from build123d import *

# Parameters (mm, degrees)
SKETCH_1_W          = 55
SKETCH_1_H          = 36.8
EXTRUDE_1_DEPTH     = 24
SKETCH_2_W          = 38
SKETCH_2_H          = 36.8
CUT_EXTRUDE_1_DEPTH = 1
CHAMFER_1_SIZE      = 0.5
CHAMFER_2_SIZE      = 0.5
SKETCH_3_W          = 7.5
SKETCH_3_H          = 36.8
CUT_EXTRUDE_2_DEPTH = 20
CHAMFER_3_SIZE      = 1.5
CHAMFER_4_SIZE      = 2
CHAMFER_5_SIZE      = 2
SKETCH_4_R          = 2.1
CUT_EXTRUDE_3_DEPTH = 20
SKETCH_5_R          = 5
EXTRUDE_2_DEPTH     = 10


with BuildPart() as part:
    # 草图1 → 凸台-拉伸1 (new body)
    with BuildSketch(Plane.XY):
        with Locations((-27.5, 18.4)):
            Rectangle(SKETCH_1_W, SKETCH_1_H)
    extrude(amount=EXTRUDE_1_DEPTH)

    # 草图2 → 切除-拉伸1 (cut)
    with BuildSketch(Plane.XY.offset(24)):
        with Locations((-27.5, 18.4)):
            Rectangle(SKETCH_2_W, SKETCH_2_H)
    extrude(amount=-CUT_EXTRUDE_1_DEPTH, mode=Mode.SUBTRACT)

    # 倒角1
    chamfer_1_edges = [part.edges().sort_by_distance(p)[0] for p in [
        (-46.5, 18.4, 24),
        (-8.5, 18.4, 24),
    ]]
    chamfer(chamfer_1_edges, length=CHAMFER_1_SIZE)

    # 倒角2
    chamfer_2_edges = [part.edges().sort_by_distance(p)[0] for p in [
        (-27.5, 36.8, 23),
        (-27.5, 0, 23),
    ]]
    chamfer(chamfer_2_edges, length=CHAMFER_2_SIZE)

    # 草图3 → 切除-拉伸2 (cut)
    with BuildSketch(Plane(origin=(0, 0, 0), x_dir=(-1, 0, 0), z_dir=(0, 0, -1))):
        with Locations((3.75, 18.4)):
            Rectangle(SKETCH_3_W, SKETCH_3_H)
        with Locations((51.25, 18.4)):
            Rectangle(SKETCH_3_W, SKETCH_3_H)
    extrude(amount=-CUT_EXTRUDE_2_DEPTH, mode=Mode.SUBTRACT)

    # 倒角3
    chamfer_3_edges = [part.edges().sort_by_distance(p)[0] for p in [
        (-27.5, 0, 0),
        (-27.5, 36.8, 0),
        (-7.5, 18.4, 0),
        (-47.5, 18.4, 0),
    ]]
    chamfer(chamfer_3_edges, length=CHAMFER_3_SIZE)

    # 倒角4
    chamfer_4_edges = [part.edges().sort_by_distance(p)[0] for p in [
        (-7.5, 36.8, 10.75),
        (-7.5, 0, 10.75),
        (-47.5, 0, 10.75),
        (-47.5, 36.8, 10.75),
    ]]
    chamfer(chamfer_4_edges, length=CHAMFER_4_SIZE)

    # 倒角5
    chamfer_5_edges = [part.edges().sort_by_distance(p)[0] for p in [
        (0, 0, 22),
        (-55, 0, 22),
        (-55, 36.8, 22),
        (0, 36.8, 22),
    ]]
    chamfer(chamfer_5_edges, length=CHAMFER_5_SIZE)

    # 草图4 → 切除-拉伸3 (cut)
    with BuildSketch(Plane(origin=(0, 0, 20), x_dir=(-1, 0, 0), z_dir=(0, 0, -1))):
        with Locations((3.55, 18.4)):
            Circle(SKETCH_4_R)
        with Locations((51.45, 32.75)):
            Circle(SKETCH_4_R)
        with Locations((51.45, 4.05)):
            Circle(SKETCH_4_R)
    extrude(amount=-CUT_EXTRUDE_3_DEPTH, mode=Mode.SUBTRACT)

    # 草图5 → 凸台-拉伸2 (add)
    with BuildSketch(Plane.ZY.offset(47.5)):
        with Locations(Location((10, 18.4, 0), (0, 0, 90))):
            Circle(SKETCH_5_R)
    extrude(amount=EXTRUDE_2_DEPTH)


solid = part.part
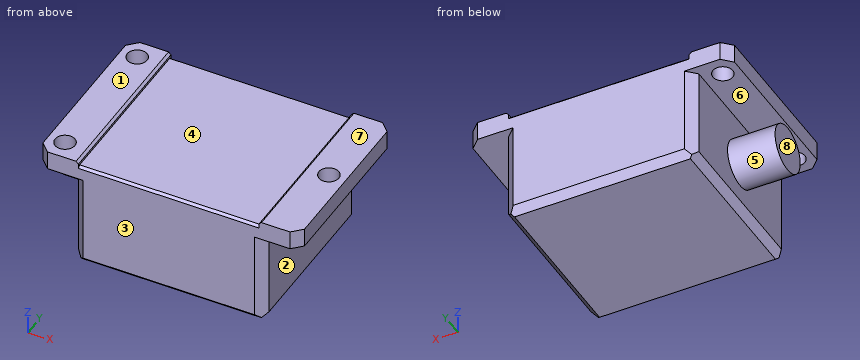
The listing builds one solid part. Answer for the finished solid, in the listing's coordinates (mm). Face numbers are marked on the shaded views. A direction names the side the tool comes from. Coordinates: 2 decimals unless noted, no trailing zeros. Loops run counter-clockwise (first coordinate to the right, second up) from the corner with the lowest first, then second, coordinate; pieces in that order, holes last. Notation, with made-up numbers: (8, -6) -> (14, -6) arc R18 cw to (14, 22) -> close; hole circle Ø1 at (-31, -35). An arc over 180 degrees is marked (long way). Answer in a Markdown table with one row per item. Add a question column.
1. The part is cut by section D-D, the plane y = 9.5. Write down the section's boundary in (x, z), then the cut area to 4 significant figures.
2. Determine the mould class of the marked faces 6, 7 and 8 for opening direction Z: +Z half, -Z half, draft (parallel to the pull), parting line (faces both ways), or undercut.
3. The part is cut by section A-A, the plane y = 18.4. Write down the section's boundary in (x, z).
4. Flat-ended cylindrical pins translate along their axes: P1, Ø4, axis at y = 18, z = 13, coming from the +X side; P2, Ø3, axis at y = 15.5, z = 21.5, coming from the -X side; P3, Ø1, axis at y = 8, z = 16.5, coming from the -X side; P4, Ø2.5, axis at x = -51.45, y = 4.05, coming from the +Z side. Find the tip coordinate at first contact, or state that the pin passes through.
5. For the marked faces 1, 2, 3, 4 and 5, determine the directions among +Z, -Z, +X, -X, +Y, -Y from which every point of the face is accessible in a straight line to the end or side of a thin tool.
6. Consider line 1 (Y direction, x = -3.55, z = 21.55); line 2 (Y direction, x = -51.45, z = 21.2); line 3 (Z direction, x = -13, y = 14). Determine where each line is inside the solid, lowest interval first. Write a range as [from, to].
7. The part is cut by section C-C, the plane x = -3.55. Write down the section's boundary in (y, z).
8. The part is cut by section B-B, the plane x = -51.45. Write down the section's boundary in (y, z), then the cut area to 3 significant figures.
Answer below:
| question | item | result |
|---|---|---|
| 1 | outline | (-55, 20) -> (-47.5, 20) -> (-47.5, 1.5) -> (-46, 0) -> (-9, 0) -> (-7.5, 1.5) -> (-7.5, 20) -> (0, 20) -> (0, 24) -> (-8, 24) -> (-8.5, 23.5) -> (-8.5, 23) -> (-46.5, 23) -> (-46.5, 23.5) -> (-47, 24) -> (-55, 24) -> close |
| 1 | area | 979.5 mm2 |
| 2 | face 6 | undercut |
| 2 | face 7 | +Z half |
| 2 | face 8 | draft |
| 3 | outline | (-57.5, 5) -> (-47.5, 5) -> (-47.5, 1.5) -> (-46, 0) -> (-9, 0) -> (-7.5, 1.5) -> (-7.5, 20) -> (-5.65, 20) -> (-5.65, 24) -> (-8, 24) -> (-8.5, 23.5) -> (-8.5, 23) -> (-46.5, 23) -> (-46.5, 23.5) -> (-47, 24) -> (-55, 24) -> (-55, 20) -> (-47.5, 20) -> (-47.5, 15) -> (-57.5, 15) -> close; (-1.45, 20) -> (0, 20) -> (0, 24) -> (-1.45, 24) -> close |
| 4 | P1 | x = -7.5 |
| 4 | P2 | x = -55 |
| 4 | P3 | x = -47.5 |
| 4 | P4 | through |
| 5 | face 1 | +Z, +X, -X, +Y, -Y |
| 5 | face 2 | -Z, +X, +Y, -Y |
| 5 | face 3 | +Z, -Z, +X, -X, -Y |
| 5 | face 4 | +Z, +Y, -Y |
| 5 | face 5 | -X |
| 6 | line 1 | [0, 16.3], [20.5, 36.8] |
| 6 | line 2 | [0, 1.95], [6.15, 30.65], [34.85, 36.8] |
| 6 | line 3 | [0, 23] |
| 7 | outline | (0, 20) -> (16.3, 20) -> (16.3, 24) -> (0, 24) -> close; (20.5, 20) -> (36.8, 20) -> (36.8, 24) -> (20.5, 24) -> close |
| 8 | outline | (0, 20) -> (1.95, 20) -> (1.95, 24) -> (0, 24) -> close; (6.15, 20) -> (30.65, 20) -> (30.65, 24) -> (6.15, 24) -> close; circle Ø10 at (18.4, 10); (34.85, 20) -> (36.8, 20) -> (36.8, 24) -> (34.85, 24) -> close |
| 8 | area | 192 mm2 |
